Could you check a few things on this model? Use its own coordinates, in mm. A direction names the side the tool comes from. Coordinates: 2 decimals unless noted, no trailing zeros. Order: outer loops, then holes, each group sorted by start corner. A loop starts at its lowest first (then second) coordinate and runs counter-clockwise, first axis right, second up. Notation, with made-up numbers: (50.5, -29) -> (77.5, -29) arc R11 cw to (77.5, -9) -> close; hole circle Ø9 at (87, 56). An arc over 180 degrees is marked (long way). Use a Markdown table: item, result. Add a question column.
1) If we section it at C-C (y = 94.5): Write out the boundary of the cut face in (x, z), plus the area to 3 significant figures.
2) If I drill on L1, parallel to Y at x = 255, z = 1.3; L2, parallel to X at y = 4.5, z = 2.8; L3, parallel to Y at x = 15.3, z = 2.6, over which ranges is the centre line in solid material (lowest first)? Write a range as [from, to].
3) If we section it at D-D (z = 1.4): Give the number of separate pieces and of enclosed holes in the cut face, plus the area to 3 significant figures.
4) If we section it at A-A (y = -28): Write out the boundary of the cut face in (x, z).
5) Thinking about a two-plate mould opening in Y: for faces 4 (the cylindrical face through (234.26, -14.99, 2.54)), 5 (the flat face through (-22, -21, 3)), 6 (the flat face through (200, 65.2, 2)), which applies, +Y half, -Y half, draft (parallel to the pull), parting line (faces both ways), or undercut?
6) Will these pins go through, and if not, where does the flat tip stop? pin 1 Ø5 at (x, y) = (46, 55.7) entering from +Z; pin 2 Ø2.5 at (x, y) = (236.99, -19.8) entering from +Z; pin 3 Ø1 at (y, z) = (40, 1) entering from -X; pin 4 Ø3 at (x, z) = (201.5, 1.5) entering from +Y.
7) If we section it at B-B (x = 174.5): Write out the boundary of the cut face in (y, z), plus the area to 3 significant figures.
8) Which directions (+Z, -Z, +X, -X, +Y, -Y) give clear straight access to the entire face, cutting with the end or side of a thin tool? Please do faces 1 (the flat face through (117, 105.2, 3)), 2 (the flat face through (0, 33, 2)), 3 (the flat face through (247, 0, 2)).
```python
from build123d import *

# Parameters (mm, degrees)
BOSS_EXTRU_2_DEPTH       = 5
ESQUISSE2_R              = 1.5
ENL_V_MAT_EXTRU_1_DEPTH  = 14
ESQUISSE3_R              = 1.5
ENL_V_MAT_EXTRU_2_DEPTH  = 32
ESQUISSE4_R              = 1.5
ENL_V_MAT_EXTRU_3_DEPTH  = 293.72553698
ESQUISSE5_R              = 1.500580152
ENL_V_MAT_EXTRU_4_DEPTH  = 293.72553698
ESQUISSE6_R              = 1.5
ENL_V_MAT_EXTRU_5_DEPTH  = 293.72553698
ESQUISSE7_R              = 1.5
ENL_V_MAT_EXTRU_6_DEPTH  = 293.72553698
ESQUISSE8_W              = 88
ESQUISSE8_H              = 33
ENL_V_MAT_EXTRU_7_DEPTH  = 293.72553698
ESQUISSE9_R              = 1.5
ESQUISSE9_R_2            = 1.507357215
ENL_V_MAT_EXTRU_8_DEPTH  = 279.668333328
ESQUISSE10_W             = 280
ESQUISSE10_H             = 4
BOSS_EXTRU_3_DEPTH       = 5
ESQUISSE12_R             = 16
ENL_V_MAT_EXTRU_10_DEPTH = 279.668333328
ESQUISSE13_R             = 1.5
ENL_V_MAT_EXTRU_11_DEPTH = 279.668333328


with BuildPart() as part:
    # Esquisse1 → Boss.-Extru.2 (new body)
    with BuildSketch(Plane.XY):
        Polygon((-22, -37), (258, -37), (258, 0), (236, 0), (236, 65.2), (162, 65.2), (162, 138.2), (74, 138.2), (74, 65.2), (0, 65.2), (0, 0), (-22, 0), align=None)
    extrude(amount=BOSS_EXTRU_2_DEPTH)

    # Esquisse2 → Enlèv. mat.-Extru.1 (cut)
    with BuildSketch(Plane.XY.offset(5)):
        with Locations((26, 55.7)):
            Circle(ESQUISSE2_R)
        with Locations((46, 55.7)):
            Circle(ESQUISSE2_R)
        with Locations((6, 55.7)):
            Circle(ESQUISSE2_R)
        with Locations((6, 45.7)):
            Circle(ESQUISSE2_R)
        with Locations((-4, -4.3)):
            Circle(ESQUISSE2_R)
        with Locations((-14, -4.3)):
            Circle(ESQUISSE2_R)
        with Locations((-4, -19.3)):
            Circle(ESQUISSE2_R)
        with Locations((-14, -19.3)):
            Circle(ESQUISSE2_R)
    extrude(amount=-ENL_V_MAT_EXTRU_1_DEPTH, mode=Mode.SUBTRACT)

    # Esquisse3 → Enlèv. mat.-Extru.2 (cut)
    with BuildSketch(Plane.XY.offset(5)):
        with Locations((132.331204837, 62.002269793)):
            Circle(ESQUISSE3_R)
    extrude(amount=-ENL_V_MAT_EXTRU_2_DEPTH, mode=Mode.SUBTRACT)

    # Esquisse4 → Enlèv. mat.-Extru.3 (cut, through all)
    with BuildSketch(Plane(origin=(0, 0, 0), x_dir=(-1, 0, 0), z_dir=(0, 0, -1))):
        with Locations((-190, 51.7)):
            Circle(ESQUISSE4_R)
        with Locations((-190, 41.7)):
            Circle(ESQUISSE4_R)
    extrude(amount=-ENL_V_MAT_EXTRU_3_DEPTH, mode=Mode.SUBTRACT)

    # Esquisse5 → Enlèv. mat.-Extru.4 (cut, through all)
    with BuildSketch(Plane.XY.offset(5)):
        with Locations((46, 45.7)):
            Circle(ESQUISSE5_R)
    extrude(amount=-ENL_V_MAT_EXTRU_4_DEPTH, mode=Mode.SUBTRACT)

    # Esquisse6 → Enlèv. mat.-Extru.5 (cut, through all)
    with BuildSketch(Plane.XY.offset(5)):
        with Locations((245, -4.3)):
            Circle(ESQUISSE6_R)
        with Locations((255, -4.3)):
            Circle(ESQUISSE6_R)
        with Locations((255, -19.3)):
            Circle(ESQUISSE6_R)
        with Locations((245, -19.3)):
            Circle(ESQUISSE6_R)
    extrude(amount=-ENL_V_MAT_EXTRU_5_DEPTH, mode=Mode.SUBTRACT)

    # Esquisse7 → Enlèv. mat.-Extru.6 (cut, through all)
    with BuildSketch(Plane(origin=(0, 0, 0), x_dir=(-1, 0, 0), z_dir=(0, 0, -1))):
        with Locations((-15.3, 28.6)):
            Circle(ESQUISSE7_R)
        with Locations((-2.6, 15.9)):
            Circle(ESQUISSE7_R)
        with Locations((-15.3, 3.2)):
            Circle(ESQUISSE7_R)
        with Locations((-28, 15.9)):
            Circle(ESQUISSE7_R)
        with Locations((-208, 15.9)):
            Circle(ESQUISSE7_R)
        with Locations((-220.7, 3.2)):
            Circle(ESQUISSE7_R)
        with Locations((-233.4, 15.9)):
            Circle(ESQUISSE7_R)
        with Locations((-220.7, 28.6)):
            Circle(ESQUISSE7_R)
    extrude(amount=-ENL_V_MAT_EXTRU_6_DEPTH, mode=Mode.SUBTRACT)

    # Esquisse8 → Enlèv. mat.-Extru.7 (cut, through all)
    with BuildSketch(Plane.XY.offset(5)):
        with Locations((118, 121.7)):
            Rectangle(ESQUISSE8_W, ESQUISSE8_H)
    extrude(amount=-ENL_V_MAT_EXTRU_7_DEPTH, mode=Mode.SUBTRACT)

    # Esquisse9 → Enlèv. mat.-Extru.8 (cut, through all)
    with BuildSketch(Plane.XY.offset(5)):
        with Locations((182.7, -20.4)):
            Circle(ESQUISSE9_R)
        with Locations((157.7, -20.4)):
            Circle(ESQUISSE9_R)
        with Locations((157.7, 9.6)):
            Circle(ESQUISSE9_R)
        with Locations((182.7, 9.6)):
            Circle(ESQUISSE9_R_2)
        with Locations((78.424217253, -21.095134328)):
            Circle(ESQUISSE9_R)
        with Locations((53.424217253, -21.095134328)):
            Circle(ESQUISSE9_R)
        with Locations((78.424217253, 8.904865672)):
            Circle(ESQUISSE9_R)
        with Locations((53.424217253, 8.904865672)):
            Circle(ESQUISSE9_R)
    extrude(amount=-ENL_V_MAT_EXTRU_8_DEPTH, mode=Mode.SUBTRACT)

    # Esquisse10 → Boss.-Extru.3 (add)
    with BuildSketch(Plane.XY.offset(5)):
        with Locations((118, -39)):
            Rectangle(ESQUISSE10_W, ESQUISSE10_H)
    extrude(amount=-BOSS_EXTRU_3_DEPTH)

    # Esquisse12 → Enlèv. mat.-Extru.10 (cut, through all)
    with BuildSketch(Plane.XY.offset(5)):
        with Locations((20.424217253, -19.8)):
            Circle(ESQUISSE12_R)
        with Locations((219, -19.8)):
            Circle(ESQUISSE12_R)
    extrude(amount=-ENL_V_MAT_EXTRU_10_DEPTH, mode=Mode.SUBTRACT)

    # Esquisse13 → Enlèv. mat.-Extru.11 (cut, through all)
    with BuildSketch(Plane.XY.offset(5)):
        with Locations((2.383457441, -19.8)):
            Circle(ESQUISSE13_R)
        with Locations((20.424217253, -1.741178451)):
            Circle(ESQUISSE13_R)
        with Locations((38.478848473, -20.040125082)):
            Circle(ESQUISSE13_R)
        with Locations((20.424217253, -37.870789792)):
            Circle(ESQUISSE13_R)
        with Locations((218.965275761, -1.741178451)):
            Circle(ESQUISSE13_R)
        with Locations((236.986339902, -19.8)):
            Circle(ESQUISSE13_R)
        with Locations((200.994611176, -19.8)):
            Circle(ESQUISSE13_R)
        with Locations((218.965275761, -37.870789792)):
            Circle(ESQUISSE13_R)
    extrude(amount=-ENL_V_MAT_EXTRU_11_DEPTH, mode=Mode.SUBTRACT)


solid = part.part
```
Answer sheet:
| question | item | result |
|---|---|---|
| 1 | outline | (74, 0) -> (162, 0) -> (162, 5) -> (74, 5) -> close |
| 1 | area | 440 mm2 |
| 2 | L1 | [-41, -20.8], [-17.8, -5.8], [-2.8, 0] |
| 2 | L2 | [0, 14.55], [16.05, 219.95], [221.45, 236] |
| 2 | L3 | [-41, -34.96], [-4.64, 1.7], [4.7, 27.1], [30.1, 65.2] |
| 3 | separate pieces | 1 |
| 3 | enclosed holes | 42 |
| 3 | area | 28,500 mm2 |
| 4 | outline | (-22, 0) -> (6.69, 0) -> (6.69, 5) -> (-22, 5) -> close; (34.16, 0) -> (205.26, 0) -> (205.26, 5) -> (34.16, 5) -> close; (232.74, 0) -> (258, 0) -> (258, 5) -> (232.74, 5) -> close |
| 5 | face 4 | undercut |
| 5 | face 5 | draft |
| 5 | face 6 | +Y half |
| 6 | pin 1 | z = 5 |
| 6 | pin 2 | through |
| 6 | pin 3 | x = 0 |
| 6 | pin 4 | y = 65.2 |
| 7 | outline | (-41, 0) -> (65.2, 0) -> (65.2, 5) -> (-41, 5) -> close |
| 7 | area | 531 mm2 |
| 8 | face 1 | +Z, -Z, +X, -X, +Y |
| 8 | face 2 | +Z, -Z, -X, +Y |
| 8 | face 3 | +Z, -Z, +X, +Y |
